Here's how the part is built. I have some questions about the finished solid (model axes, mm). Coordinates: 2 decimals unless noted, no trailing zeros. Write each loop counter-clockwise with the first axis right and the second up, starting at its lowest first coordinate (ties: lowest second). Pieces come first, ordered by that corner, then holes. Notation, with made-up numbers: (-32, -1) -> (24, -1) arc R35 ccw to (24, 36) -> close; hole circle Ø5 at (-29.75, 31). An arc over 180 degrees is marked (long way). Put each result on its own line as item: value.
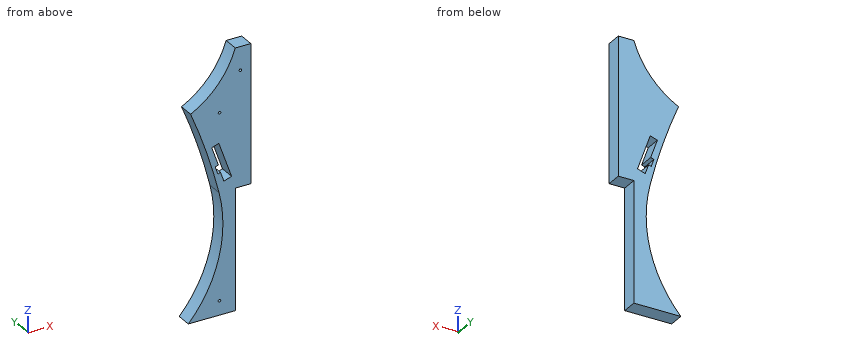
```python
from build123d import *

# Parameters (mm, degrees)
BOSS_EXTRUDE1_DEPTH              = 19.05
CUT_EXTRUDE2_DEPTH               = 328.154074659
F_1_8_0_125_DIAMETER_HOLE1_D     = 3.175
F_1_8_0_125_DIAMETER_HOLE1_DEPTH = 11.1252
F_1_8_0_125_DIAMETER_HOLE1_TIP   = 0.953866233


with BuildPart() as part:
    # Sketch1 → Boss-Extrude1 (new body)
    with BuildSketch(Plane(origin=(0, 0, 0), x_dir=(1, 0, 0), z_dir=(0, 1, 0))):
        with BuildLine():
            Line((0, 169.388632852), (0, 0))
            Line((0, 0), (-19.05, 0))
            ThreePointArc((-19.05, 0), (-39.88804557, 37.868270719), (-73.722410895, 64.765590165))
            ThreePointArc((-73.722410895, 64.765590165), (-54.193392954, 116.375662835), (-38.876501861, 169.388632852))
            ThreePointArc((-38.876501861, 169.388632852), (-39.194658591, 248.155900408), (-76.554791267, 317.5))
            Line((-76.554791267, 317.5), (-19.05, 317.5))
            Line((-19.05, 317.5), (-19.05, 169.388632852))
            Line((-19.05, 169.388632852), (0, 169.388632852))
        make_face()
    extrude(amount=BOSS_EXTRUDE1_DEPTH)

    # Sketch2 → Cut-Extrude2 (cut, through all)
    with BuildSketch(Plane(origin=(0, 19.05, 0), x_dir=(1, 0, 0), z_dir=(0, 1, 0))):
        Polygon((-39.164098049, 109.561842364), (-23.543572116, 153.825683885), (-32.944847981, 157.143355113), (-37.133143759, 145.274992843), (-40.27089443, 146.38229203), (-43.588565658, 136.981016166), (-39.696317688, 135.607458014), (-47.810876614, 112.613254626), align=None)
    extrude(amount=-CUT_EXTRUDE2_DEPTH, mode=Mode.SUBTRACT)

    # 1/8 (0.125) Diameter Hole1
    with Locations(Plane(origin=(0, 0, 0), x_dir=(-1, 0, 0), z_dir=(0, -1, 0))):
        with Locations((12.7, 28.575), (38.363219465, 73.025), (38.363219465, 300.0375)):
            Hole(F_1_8_0_125_DIAMETER_HOLE1_D / 2, depth=F_1_8_0_125_DIAMETER_HOLE1_DEPTH)
            with Locations((0, 0, -(F_1_8_0_125_DIAMETER_HOLE1_DEPTH + F_1_8_0_125_DIAMETER_HOLE1_TIP / 2))):  # 118° drill point
                Cone(0, F_1_8_0_125_DIAMETER_HOLE1_D / 2, F_1_8_0_125_DIAMETER_HOLE1_TIP, mode=Mode.SUBTRACT)


solid = part.part
```
Item 1: Imagine slicing it at C-C on x = -71. Write out the boundary of the cut face in (y, z).
Output:
outline: (0, -317.5) -> (19.05, -317.5) -> (19.05, -311.08) -> (0, -311.08) -> close; (0, -71.26) -> (19.05, -71.26) -> (19.05, -63.32) -> (0, -63.32) -> close
Item 2: Please list where these lines run through material, in increasing order: line 1 along X through (y, z) = (8.5, -165); line 2 along Z through (x, y) = (-4, 17.75); line 3 along X through (y, z) = (12.25, -138.5). Write a range as from..to.
Output:
line 1: x = -39.97..0
line 2: z = -169.39..0
line 3: x = -47.24..-43.05, -28.95..0
Item 3: Imagine slicing it at B-B on x = -51. Write out the boundary of the cut face in (y, z), then the cut area to 3 significant figures.
Output:
outline: (0, -317.5) -> (19.05, -317.5) -> (19.05, -280.08) -> (0, -280.08) -> close; (0, -126.21) -> (19.05, -126.21) -> (19.05, -49.25) -> (0, -49.25) -> close
area: 2,180 mm²
Item 4: Imagine slicing it at D-D on z = -90. Write out the boundary of the cut face in (x, y), then the cut area to 3 significant figures.
Output:
outline: (-63.58, 0) -> (0, 0) -> (0, 19.05) -> (-63.58, 19.05) -> close
area: 1,210 mm²
Item 5: For P1, Ø5, axis at y = 13, z = -243.5, coming from the -X side; P2, Ø1.5, axis at y = 10, z = -68, coming from the -X side; P3, Ø3, axis at x = -12.7, z = -28.575, coming from the -Y side, each with a flat end and sliding along its axis, tell me the tip position at first contact or that it passes through.
Output:
P1: stops at x = -38.66
P2: stops at x = -72.67
P3: stops at y = 11.18
